```python
from build123d import *

# Parameters (mm, degrees)
F1_W     = 1.6002
F1_H     = 1.6002
F1_W_2   = 1.142379
F1_H_2   = 10.922
F1_W_3   = 3.302
F1_H_3   = 2.54
F2_DEPTH = 1.524
F3_R     = 3.175


with BuildPart() as f2:
    # F1 (on Front) → F2 (new body)
    with BuildSketch(Plane.XZ):
        with BuildLine():
            ThreePointArc((-13.103278, 47.625), (-7.439488, 43.360512), (-3.175, 37.696722))
            Line((-3.175, 37.696722), (-3.175, 47.625))
            Line((-3.175, 47.625), (-13.103278, 47.625))
        make_face()
        with BuildLine():
            ThreePointArc((-47.625, 13.103278), (-43.360512, 7.439488), (-37.696722, 3.175))
            Line((-37.696722, 3.175), (-13.103278, 3.175))
            ThreePointArc((-13.103278, 3.175), (-7.439488, 7.439488), (-3.175, 13.103278))
            Line((-3.175, 13.103278), (-3.175, 37.696722))
            ThreePointArc((-3.175, 37.696722), (-7.439488, 43.360512), (-13.103278, 47.625))
            Line((-13.103278, 47.625), (-37.696722, 47.625))
            ThreePointArc((-37.696722, 47.625), (-43.360512, 43.360512), (-47.625, 37.696722))
            Line((-47.625, 37.696722), (-47.625, 13.103278))
        make_face()
        with Locations((-40.399718, 10.952067)):
            Rectangle(F1_W, F1_H, mode=Mode.SUBTRACT)
        with BuildLine():
            ThreePointArc((-34.914493, 19.881328), (-36.500967, 19.132292), (-37.482908, 17.678419))
            ThreePointArc((-37.482908, 17.678419), (-37.822793, 15.612967), (-37.482908, 13.547515))
            ThreePointArc((-37.482908, 13.547515), (-36.500967, 12.093642), (-34.914493, 11.344606))
            Line((-34.914493, 11.344606), (-34.914493, 10.188754))
            ThreePointArc((-34.914493, 10.188754), (-37.168718, 11.162006), (-38.565638, 13.181256))
            ThreePointArc((-38.565638, 13.181256), (-38.965793, 15.612967), (-38.565638, 18.044678))
            ThreePointArc((-38.565638, 18.044678), (-37.168718, 20.063928), (-34.914493, 21.037181))
            Line((-34.914493, 21.037181), (-34.914493, 19.881328))
        make_face(mode=Mode.SUBTRACT)
        with BuildLine():
            ThreePointArc((-30.120348, 18.044678), (-29.720193, 15.612967), (-30.120348, 13.181256))
            ThreePointArc((-30.120348, 13.181256), (-31.517268, 11.162006), (-33.771493, 10.188754))
            Line((-33.771493, 10.188754), (-33.771493, 11.344606))
            ThreePointArc((-33.771493, 11.344606), (-32.185019, 12.093642), (-31.203077, 13.547515))
            ThreePointArc((-31.203077, 13.547515), (-30.863193, 15.612967), (-31.203077, 17.678419))
            ThreePointArc((-31.203077, 17.678419), (-32.185019, 19.132292), (-33.771493, 19.881328))
            Line((-33.771493, 19.881328), (-33.771493, 21.037181))
            ThreePointArc((-33.771493, 21.037181), (-31.517268, 20.063928), (-30.120348, 18.044678))
        make_face(mode=Mode.SUBTRACT)
        with Locations((-27.294804, 15.612967)):
            Rectangle(F1_W_2, F1_H_2, mode=Mode.SUBTRACT)
        with BuildLine():
            Line((-23.058243, 14.716427), (-20.218135, 10.151967))
            Line((-20.218135, 10.151967), (-21.564335, 10.151967))
            Line((-21.564335, 10.151967), (-24.251414, 14.470487))
            add(Edge.make_bspline(
                [(-25.580614, 14.470296), (-25.412167, 14.47032), (-24.9691, 14.470384), (-24.526034, 14.470447), (-24.251414, 14.470487)],
                knots=[1.142379, 1.142379, 1.142379, 1.142379, 1.647719, 2.471579, 2.471579, 2.471579, 2.471579], degree=3))
            Line((-25.580614, 14.470296), (-25.580614, 15.613296))
            Line((-25.580614, 15.613296), (-24.2627, 15.613485))
            ThreePointArc((-24.2627, 15.613485), (-22.151123, 17.795615), (-24.309993, 19.930967))
            Line((-24.309993, 19.930967), (-25.580614, 19.930967))
            Line((-25.580614, 19.930967), (-25.580614, 21.073967))
            Line((-25.580614, 21.073967), (-24.309993, 21.073967))
            ThreePointArc((-24.309993, 21.073967), (-21.070194, 18.409858), (-23.058243, 14.716427))
        make_face(mode=Mode.SUBTRACT)
        with BuildLine():
            ThreePointArc((-17.767223, 13.547515), (-15.565822, 11.430607), (-12.567683, 12.012518))
            Line((-12.567683, 12.012518), (-12.567683, 14.469967))
            Line((-12.567683, 14.469967), (-14.627307, 14.469967))
            Line((-14.627307, 14.469967), (-14.627307, 15.612967))
            Line((-14.627307, 15.612967), (-11.424683, 15.612967))
            Line((-11.424683, 15.612967), (-11.424683, 11.508976))
            ThreePointArc((-11.424683, 11.508976), (-15.606715, 10.260892), (-18.849952, 13.181256))
            ThreePointArc((-18.849952, 13.181256), (-19.250107, 15.612967), (-18.849952, 18.044678))
            ThreePointArc((-18.849952, 18.044678), (-15.610848, 20.96411), (-11.430582, 19.72304))
            Line((-11.430582, 19.72304), (-12.141509, 18.808992))
            ThreePointArc((-12.141509, 18.808992), (-15.280389, 19.865993), (-17.767223, 17.678419))
            ThreePointArc((-17.767223, 17.678419), (-18.107107, 15.612967), (-17.767223, 13.547515))
        make_face(mode=Mode.SUBTRACT)
        with BuildLine():
            Line((-30.890982, 40.37965), (-30.890982, 29.35605))
            ThreePointArc((-30.890982, 29.35605), (-33.927344, 24.913031), (-39.169881, 26.127817))
            Line((-39.169881, 26.127817), (-37.674255, 27.503363))
            ThreePointArc((-37.674255, 27.503363), (-34.665555, 26.806195), (-32.922982, 29.35605))
            Line((-32.922982, 29.35605), (-32.922982, 40.37965))
            Line((-32.922982, 40.37965), (-30.890982, 40.37965))
        make_face(mode=Mode.SUBTRACT)
        with Locations((-25.4, 44.831)):
            Rectangle(F1_W_3, F1_H_3, mode=Mode.SUBTRACT)
        Polygon((-28.856911, 40.37965), (-26.778254, 40.37965), (-24.283081, 28.802234), (-21.238982, 39.617483), (-18.698982, 39.617483), (-15.654884, 28.802234), (-13.159711, 40.37965), (-11.081054, 40.37965), (-14.484654, 24.5872), (-16.57946, 24.5872), (-19.968982, 36.629689), (-23.358505, 24.5872), (-25.453311, 24.5872), align=None, mode=Mode.SUBTRACT)
        with BuildLine():
            ThreePointArc((-3.175, 13.103278), (-7.439488, 7.439488), (-13.103278, 3.175))
            Line((-13.103278, 3.175), (-3.175, 3.175))
            Line((-3.175, 3.175), (-3.175, 13.103278))
        make_face()
        with BuildLine():
            Line((-47.625, 47.625), (-47.625, 37.696722))
            ThreePointArc((-47.625, 37.696722), (-43.360512, 43.360512), (-37.696722, 47.625))
            Line((-37.696722, 47.625), (-47.625, 47.625))
        make_face()
        with BuildLine():
            Line((-47.625, 3.175), (-37.696722, 3.175))
            ThreePointArc((-37.696722, 3.175), (-43.360512, 7.439488), (-47.625, 13.103278))
            Line((-47.625, 13.103278), (-47.625, 3.175))
        make_face()
    extrude(amount=F2_DEPTH)

    # F3
    f3_edges = [f2.edges().sort_by_distance(p)[0] for p in [
        (-47.625, -0.762, 47.625),
        (-3.175, -0.762, 47.625),
        (-3.175, -0.762, 3.175),
        (-47.625, -0.762, 3.175),
    ]]
    fillet(f3_edges, radius=F3_R)


solid = f2.part
```
Geometry check sheet. Reference: the model listing, model coordinates, mm. A direction names the side the tool comes from. Coordinates: 2 decimals unless noted, no trailing zeros. Write each loop counter-clockwise with the first axis right and the second up, starting at its lowest first coordinate (ties: lowest second). Pieces come first, ordered by that corner, then holes. Notation, with made-up numbers: M 38.25,-39 L 62.25,-39 A13 ccw 62.25,-15 Z; hole C -26.5,-31 d7. An arc over 180 degrees is marked long. Answer as a JSON object with one key per item and string values.
1. Section check C-C, the plane z = 36. Enter the section's corners in (x, y) (3 decimals), plus the area to 3 significant figures.
Answers below:
{"outline": "M -47.625,-1.524 L -32.923,-1.524 L -32.923,0 L -47.625,0 Z; M -30.891,-1.524 L -27.913,-1.524 L -27.913,0 L -30.891,0 Z; M -25.834,-1.524 L -22.257,-1.524 L -22.257,0 L -25.834,0 Z; M -20.146,-1.524 L -19.792,-1.524 L -19.792,0 L -20.146,0 Z; M -17.681,-1.524 L -14.104,-1.524 L -14.104,0 L -17.681,0 Z; M -12.025,-1.524 L -3.175,-1.524 L -3.175,0 L -12.025,0 Z", "area": "51.9 mm²"}
2. Draft check along X on faces 1 (the flat face through (-25, -1, 47.625)), 2 (the flat face through (-17.2, -0.75, 34.29)), 3 (the cylindrical face through (-4.13, -0.77, 46.72)). Enter one of: released by +X, released by -X, zero draft, split by the parting line, or undercut.
Answers below:
{"face 1": "zero draft", "face 2": "undercut", "face 3": "released by +X"}
3. Section check A-A, the plane z = 45. Enter the section's corners in (x, y).
Answers below:
{"outline": "M -47.58,-1.52 L -27.05,-1.52 L -27.05,0 L -47.58,0 Z; M -23.75,-1.52 L -3.22,-1.52 L -3.22,0 L -23.75,0 Z"}
4. Section check B-B, the plane y = -0.25. Give the number of separate pieces and of enclosed holes in the cut face, plus the area to 3 significant figures.
Answers below:
{"separate pieces": "1", "enclosed holes": "9", "area": "1,710 mm²"}
5. Tool access check on faces 4 (the flat face through (-41.2, -1, 11)), 5 (the flat face through (-47.625, -1, 26)). Record the directions out of +Z, -Z, +X, -X, +Y, -Y that give a thin tool (end or side, any length) a straight path to the whole face; none if there is none.
Answers below:
{"face 4": "+Y, -Y", "face 5": "+Z, -Z, -X, +Y, -Y"}
6. Scan lines: L1, parallel to X at y = -0.1, z = 35 (3 decimals); L2, parallel to X at y = -0.15, z = 26 (3 decimals); L3, parallel to X at y = -1.4, z = 31 (3 decimals). Record each from-to range of solid material in increasing order.
Answers below:
{"L1": "x = -47.625 to -32.923, -30.891 to -27.697, -25.619 to -22.539, -20.428 to -19.51, -17.399 to -14.319, -12.24 to -3.175", "L2": "x = -47.625 to -39.048, -32.272 to -25.758, -22.961 to -16.977, -14.18 to -3.175", "L3": "x = -47.625 to -32.923, -30.891 to -26.835, -24.757 to -23.664, -21.554 to -18.384, -16.273 to -15.181, -13.103 to -3.175"}
